Model file for the job. Use its own axes, mm. A direction names the side the tool comes from. Round coordinates to 2 decimals unless told otherwise and drop trailing zeros. Loops run counter-clockwise (first coordinate to the right, second up) from the corner with the lowest first, then second, coordinate; pieces in that order, holes last. Notation, with made-up numbers: (35.25, 35) - (49.25, 35) arc R28 cw to (49.25, 58) - close; hole circle Ø1 at (24, 46.25). An arc over 180 degrees is marked (long way). Use one line per item in the form item = value.
from build123d import *

# Parameters (mm, degrees)
SKETCH1_W           = 82
SKETCH1_H           = 73.66
BOSS_EXTRUDE1_DEPTH = 4
SKETCH2_W           = 4.88717895
SKETCH2_H           = 73.66
BOSS_EXTRUDE2_DEPTH = 25
SKETCH3_R           = 1.45
CUT_EXTRUDE1_DEPTH  = 10
SKETCH4_W           = 24.37
SKETCH4_H           = 61.062715067
CUT_EXTRUDE2_DEPTH  = 10


with BuildPart() as part:
    # Sketch1 → Boss-Extrude1 (new body)
    with BuildSketch(Plane(origin=(0, 0, 0), x_dir=(1, 0, 0), z_dir=(0, 1, 0))):
        with Locations((0.667646454, -2.157941762)):
            Rectangle(SKETCH1_W, SKETCH1_H)
    extrude(amount=BOSS_EXTRUDE1_DEPTH)

    # Sketch2 → Boss-Extrude2 (add)
    with BuildSketch(Plane(origin=(0, 4, 0), x_dir=(1, 0, 0), z_dir=(0, 1, 0))):
        with Locations((39.271911138, -2.157941762)):
            Rectangle(SKETCH2_W, SKETCH2_H)
    extrude(amount=BOSS_EXTRUDE2_DEPTH)

    # Sketch3 → Cut-Extrude1 (cut)
    with BuildSketch(Plane(origin=(0, 4, 0), x_dir=(1, 0, 0), z_dir=(0, 1, 0))):
        with Locations((-30.544050148, 9.782058238)):
            Circle(SKETCH3_R)
        with Locations((-30.544050148, -14.097941762)):
            Circle(SKETCH3_R)
    extrude(amount=-CUT_EXTRUDE1_DEPTH, mode=Mode.SUBTRACT)

    # Sketch4 → Cut-Extrude2 (cut)
    with BuildSketch(Plane(origin=(0, 4, 0), x_dir=(1, 0, 0), z_dir=(0, 1, 0))):
        with Locations((-13.885112628, -2.028636366)):
            Rectangle(SKETCH4_W, SKETCH4_H)
    extrude(amount=-CUT_EXTRUDE2_DEPTH, mode=Mode.SUBTRACT)


solid = part.part
1. Tool access for faces 1 (the flat face through (-1.7, 2, 2)), 2 (the flat face through (6, 4, 2)): list every direction of +Z, -Z, +X, -X, +Y, -Y with a clear straight run to the whole face (end or side of a thin tool).
Geometry check:
face_1 = +Y, -Y
face_2 = +Z, -Z, -X, +Y
2. Cut at D-D, the plane x = 16. Give the cut face in (y, z), plus the area to 3 significant figures.
Geometry check:
outline = (0, -34.67) - (4, -34.67) - (4, 38.99) - (0, 38.99) - close
area = 295 mm^2
3. Wall check: probe 1 along X at (y, z) = (2.25, 6.5); probe 2 along Y at (x, z) = (4, 12); probe 3 along X at (y, z) = (21.75, -18.5). Give the ranges that are in metal, low to high.
Geometry check:
probe_1 = -40.33 to -26.07, -1.7 to 41.67
probe_2 = 0 to 4
probe_3 = 36.83 to 41.72
4. Cut at A-A, the plane z = -23.5. Give the cut face in (x, y).
Geometry check:
outline = (-40.33, 0) - (-26.07, 0) - (-26.07, 4) - (-40.33, 4) - close; (-1.7, 0) - (41.67, 0) - (41.67, 4) - (41.72, 4) - (41.72, 29) - (36.83, 29) - (36.83, 4) - (-1.7, 4) - close
5. Cut at B-B, the plane x = -9.5. Give the cut face in (y, z).
Geometry check:
outline = (0, -34.67) - (4, -34.67) - (4, -28.5) - (0, -28.5) - close; (0, 32.56) - (4, 32.56) - (4, 38.99) - (0, 38.99) - close
6. Flat gauge pins, fed straight in: pin 1 (22 mm diameter, centred on x = -3.5, z = 9, fed in from +Y); pin 2 (1.2 mm diameter, centred on y = 2, z = -12, fed in from +X). Where does each tip first touch, or does it go through?
Geometry check:
pin_1 = 4
pin_2 = 41.67
7. Cut at C-C, the plane y = 9.5. Give the cut face in (x, z), plus the area to 3 significant figures.
Geometry check:
outline = (36.83, -34.67) - (41.72, -34.67) - (41.72, 38.99) - (36.83, 38.99) - close
area = 360 mm^2
